Geometry check sheet. Reference: the model listing, model coordinates, mm. A direction names the side the tool comes from. Coordinates: 2 decimals unless noted, no trailing zeros. Write each loop counter-clockwise with the first axis right and the second up, starting at its lowest first coordinate (ties: lowest second). Pieces come first, ordered by that corner, then holes. Notation, with made-up numbers: M -34,-31 L -22,-31 A17 cw -22,1 Z; hole C -15.5,2.5 d4. An arc over 180 degrees is marked long. Answer as a JSON object with one key per item and string values. Group by question number.
```python
from build123d import *

# Parameters (mm, degrees)
SKETCH2_R           = 12.5
BOSS_EXTRUDE1_DEPTH = 20
SKETCH3_R           = 14
BOSS_EXTRUDE2_DEPTH = 70
SKETCH4_R           = 16
BOSS_EXTRUDE3_DEPTH = 76
BOSS_EXTRUDE4_START = 64
SKETCH5_R           = 12.5
BOSS_EXTRUDE4_DEPTH = 64
SKETCH6_R           = 11
BOSS_EXTRUDE5_DEPTH = 53.5
SKETCH7_R           = 10
BOSS_EXTRUDE6_DEPTH = 20
CUT_EXTRUDE1_DEPTH  = 6
CUT_EXTRUDE2_DEPTH  = 6
CUT_EXTRUDE3_DEPTH  = 6
SKETCH12_W          = 1.2
SKETCH12_H          = 1.8


with BuildPart() as part:
    # Sketch2 → Boss-Extrude1 (new body)
    with BuildSketch(Plane.XY):
        Circle(SKETCH2_R)
    extrude(amount=BOSS_EXTRUDE1_DEPTH)

    # Sketch3 → Boss-Extrude2 (add)
    with BuildSketch(Plane(origin=(0, 0, 0), x_dir=(-1, 0, 0), z_dir=(0, 0, -1))):
        Circle(SKETCH3_R)
    extrude(amount=BOSS_EXTRUDE2_DEPTH)

    # Sketch4 → Boss-Extrude3 (add)
    with BuildSketch(Plane(origin=(0, 0, -70), x_dir=(-1, 0, 0), z_dir=(0, 0, -1))):
        Circle(SKETCH4_R)
    extrude(amount=BOSS_EXTRUDE3_DEPTH)

    # Sketch5 → Boss-Extrude4 (add)
    with BuildSketch(Plane(origin=(0, 0, -146), x_dir=(-1, 0, 0), z_dir=(0, 0, -1)).offset(BOSS_EXTRUDE4_START)):
        with Locations(Location((0, 0, 0), (0, 0, 180))):
            Circle(SKETCH5_R)
    extrude(amount=-BOSS_EXTRUDE4_DEPTH)

    # Sketch6 → Boss-Extrude5 (add)
    with BuildSketch(Plane(origin=(0, 0, -210), x_dir=(-1, 0, 0), z_dir=(0, 0, -1))):
        Circle(SKETCH6_R)
    extrude(amount=BOSS_EXTRUDE5_DEPTH)

    # Sketch7 → Boss-Extrude6 (add)
    with BuildSketch(Plane(origin=(0, 0, -263.5), x_dir=(-1, 0, 0), z_dir=(0, 0, -1))):
        Circle(SKETCH7_R)
    extrude(amount=BOSS_EXTRUDE6_DEPTH)

    # Sketch8 → Cut-Extrude1 (cut)
    with BuildSketch(Plane(origin=(0, 14, 0), x_dir=(1, 0, 0), z_dir=(0, 1, 0))):
        with BuildLine():
            Line((5, 63), (5, 35))
            ThreePointArc((5, 35), (0, 30), (-5, 35))
            Line((-5, 35), (-5, 63))
            ThreePointArc((-5, 63), (0, 68), (5, 63))
        make_face()
    extrude(amount=-CUT_EXTRUDE1_DEPTH, mode=Mode.SUBTRACT)

    # Sketch9 → Cut-Extrude2 (cut)
    with BuildSketch(Plane(origin=(0, 12.5, 0), x_dir=(1, 0, 0), z_dir=(0, 1, 0))):
        with BuildLine():
            Line((-5, 153), (-5, 178))
            ThreePointArc((-5, 178), (0, 183), (5, 178))
            Line((5, 178), (5, 153))
            ThreePointArc((5, 153), (0, 148), (-5, 153))
        make_face()
    extrude(amount=-CUT_EXTRUDE2_DEPTH, mode=Mode.SUBTRACT)

    # Sketch11 → Cut-Extrude3 (cut)
    with BuildSketch(Plane(origin=(0, 11, 0), x_dir=(1, 0, 0), z_dir=(0, 1, 0))):
        with BuildLine():
            Line((-5, 218), (-5, 240))
            ThreePointArc((-5, 240), (0, 245), (5, 240))
            Line((5, 240), (5, 218))
            ThreePointArc((5, 218), (0, 213), (-5, 218))
        make_face()
    extrude(amount=-CUT_EXTRUDE3_DEPTH, mode=Mode.SUBTRACT)

    # Sketch12 → Cut-Revolve1 (revolve, cut)
    with BuildSketch(Plane(origin=(0, 0, 0), x_dir=(0, 0, -1), z_dir=(1, 0, 0)), mode=Mode.PRIVATE) as cut_revolve1_sk:
        with Locations((25.4, 13.1)):
            Rectangle(SKETCH12_W, SKETCH12_H)
        with Locations((187.6, 11.6)):
            Rectangle(SKETCH12_W, SKETCH12_H)
        with Locations((249.6, 10.1)):
            Rectangle(SKETCH12_W, SKETCH12_H)
    revolve(cut_revolve1_sk.sketch.rotate(Axis((0, 0, 20.679207299), (0, 0, -1)), 90), axis=Axis((0, 0, 20.679207299), (0, 0, -1)), mode=Mode.SUBTRACT)


solid = part.part
```
1) Set-up check for faces 1 (the cylindrical face through (11.923, 3.755, 9.86)), 2 (the cylindrical face through (3.47, -15.62, -107.47)), 3 (the flat face through (-5, 8, -250.2)), 4 (the cylindrical face through (2.38, -10.74, -256.76)), 5 (the cylindrical face through (0, 10, -183)): record each of +Z, -Z, +X, -X, +Y, -Y from which the full face is reachable in a straight line by a thin tool's end or side.
2) Draft check along Z on faces 6 (the flat face through (5, 7, -229)), 7 (the flat face through (0, 0, 20)), 8 (the cylindrical face through (-12.932, -5.362, -12.226)). Enter one of: +Z half, -Z half, draft (parallel to the pull), parting line (faces both ways), or undercut.
3) Go/stop test with flat-tipped pins: pin 1 Ø2.5 at (y, z) = (8.5, -230) entering from +X; pin 2 Ø10 at (x, z) = (-1.5, -245) entering from +Y; pin 3 Ø1.5 at (x, z) = (-10, -29) entering from -Y. Record where each tip stops, or that it passes through.
4) Material ranges on probe 1 along Z at (x, y) = (-2, -13); probe 2 along Z at (x, y) = (9.5, 7.5); probe 3 along X at (y, z) = (-0.5, -268), recorded low to high. Write a range as [from, to].
5) Section check A-A (z = -81). Record the cut outline in (x, y), then the cut area to 3 significant figures.
Entries:
{
 "1": {"face 1": "+Z", "face 2": "+Z, -Z", "face 3": "none", "face 4": "-Z", "face 5": "+Y"},
 "2": {"face 6": "undercut", "face 7": "+Z half", "face 8": "draft"},
 "3": {"pin 1": "x = 8.27", "pin 2": "y = 11", "pin 3": "y = -10.51"},
 "4": {"probe 1": "[-146, -26], [-24.8, 0]", "probe 2": "[-210, -188.2], [-187, 20]", "probe 3": "[-9.99, 9.99]"},
 "5": {"outline": "C 0,0 d32", "area": "804 mm^2"}
}
